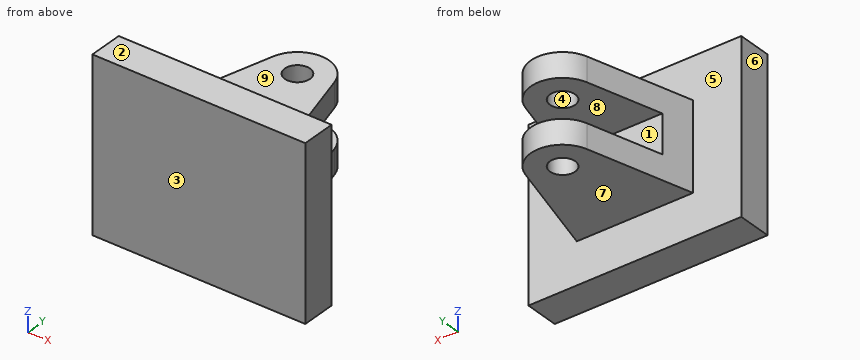
from build123d import *

# Parameters (mm, degrees)
SKETCH3_W               = 100
SKETCH3_H               = 80
BOSS_EXTRUDE2_DEPTH     = 16
BOSS_EXTRUDE3_DEPTH     = 20.5
SKETCH6_R               = 5.911815165
CUT_EXTRUDE1_DEPTH      = 109.559891304
CUT_EXTRUDE2_DEPTH      = 99.615414617
CUT_EXTRUDE2_DEPTH_BACK = 99.615414617
SKETCH8_W               = 18.118513472
SKETCH8_H               = 45.137164109


with BuildPart() as part:
    # Sketch3 → Boss-Extrude2 (new body)
    with BuildSketch(Plane(origin=(0, 0, 0), x_dir=(1, 0, 0), z_dir=(0, 1, 0))):
        Rectangle(SKETCH3_W, SKETCH3_H)
    extrude(amount=BOSS_EXTRUDE2_DEPTH)

    # Sketch5 → Boss-Extrude3 (add, symmetric)
    with BuildSketch(Plane.XY):
        with BuildLine():
            Line((-27.294131566, 16), (-14.434798789, 63.927620339))
            ThreePointArc((-14.434798789, 63.927620339), (0, 75), (14.434798789, 63.927620339))
            Line((14.434798789, 63.927620339), (27.294131566, 16))
            Line((27.294131566, 16), (-27.294131566, 16))
        make_face()
    extrude(amount=BOSS_EXTRUDE3_DEPTH, both=True)

    # Sketch6 → Cut-Extrude1 (cut, through all)
    with BuildSketch(Plane.XY.offset(20.5)):
        with Locations((0, 60.054657736)):
            Circle(SKETCH6_R)
    extrude(amount=-CUT_EXTRUDE1_DEPTH, mode=Mode.SUBTRACT)

    # Sketch8 → Cut-Extrude2 (cut, two sides: drawn at the far end of the back side and taken through both)
    with BuildSketch(Plane(origin=(0, 0, 0), x_dir=(0, 0, -1), z_dir=(1, 0, 0)).offset(-CUT_EXTRUDE2_DEPTH_BACK)):
        with Locations((0, 52.431417946)):
            Rectangle(SKETCH8_W, SKETCH8_H)
    extrude(amount=CUT_EXTRUDE2_DEPTH + CUT_EXTRUDE2_DEPTH_BACK, mode=Mode.SUBTRACT)


solid = part.part
Build history of the part. All positions in model axes, mm. Face numbers are marked on the shaded views. A direction names the side the tool comes from. Give positions to 0.01 mm unless a question says otherwise; leave off trailing zeros. Loops run counter-clockwise (first coordinate to the right, second up) from the corner with the lowest first, then second, coordinate; pieces in that order, holes last. Notation, with made-up numbers: (49.25, 76.25) - (104.25, 76.25) arc R18 cw to (104.25, 102.25) - close; hole circle Ø1 at (89, 17.25). An arc over 180 degrees is marked (long way). Write item = value, one per line. Start each with the question number.
1) Band-saw the part on A-A on x = 0. Give the cut face in (y, z), plus the area to 3 significant figures.
2) Band-saw the part on C-C on z = -18. Give the cut face in (x, y), plus the area to 3 significant figures.
3) Drop flat-ended pins along their axis: pin 1 Ø7 at (x, y) = (0, 60.05) entering from -Z; pin 2 Ø1 at (x, y) = (-11, 62) entering from +Z; pin 3 Ø6 at (y, z) = (60, -21) entering from -X; pin 4 Ø13.5 at (x, y) = (0, 60.05) entering from -Z. Give the stop position or say it passes through.
4) Band-saw the part on D-D on x = 18. Give the cut face in (y, z), plus the area to 3 significant figures.
5) Pull direction Y, two halves, no side cores. Call the marked faces 1, 2, 3 and 4: +Y half, -Y half, draft (parallel to the pull), parting line (faces both ways), or undercut.
6) Tool access for the marked faces 5, 6, 7, 8 and 9: list every direction of +Z, -Z, +X, -X, +Y, -Y with a clear straight run to the whole face (end or side of a thin tool).
7) Band-saw the part on B-B on y = 46. Give the cut face in (x, z).
8) Probe probe 1 along Y at (x, z) = (0, 13); probe 2 along Z at (x, y) = (8.5, 67.5); probe 3 along Y at (x, z) = (36, 25). List the from-to ranges inside material, lowest first. Write a range as from..to.
Final values:
q1.outline = (0, -40) - (16, -40) - (16, -20.5) - (54.14, -20.5) - (54.14, -9.06) - (29.86, -9.06) - (29.86, 9.06) - (54.14, 9.06) - (54.14, 20.5) - (16, 20.5) - (16, 40) - (0, 40) - close; (65.97, -20.5) - (75, -20.5) - (75, -9.06) - (65.97, -9.06) - close; (65.97, 9.06) - (75, 9.06) - (75, 20.5) - (65.97, 20.5) - close
q1.area = 2,610 mm²
q2.outline = (-50, 0) - (50, 0) - (50, 16) - (27.29, 16) - (14.43, 63.93) arc R14.95 ccw to (-14.43, 63.93) - (-27.29, 16) - (-50, 16) - close; hole circle Ø11.82 at (0, 60.05)
q2.area = 3,730 mm²
q3.pin_1 = through
q3.pin_2 = 20.5
q3.pin_3 = -16.28
q3.pin_4 = -20.5
q4.outline = (0, -40) - (16, -40) - (16, -20.5) - (50.64, -20.5) - (50.64, -9.06) - (29.86, -9.06) - (29.86, 9.06) - (50.64, 9.06) - (50.64, 20.5) - (16, 20.5) - (16, 40) - (0, 40) - close
q4.area = 2,320 mm²
q5.face_1 = +Y half
q5.face_2 = draft
q5.face_3 = -Y half
q5.face_4 = undercut
q6.face_5 = +Y
q6.face_6 = +Z, -Z, -X, +Y, -Y
q6.face_7 = -Z, +X, -X, +Y
q6.face_8 = +X, -X, +Y
q6.face_9 = +Z, +X, -X, +Y
q7.outline = (-19.24, -20.5) - (19.24, -20.5) - (19.24, -9.06) - (-19.24, -9.06) - close; (-19.24, 9.06) - (19.24, 9.06) - (19.24, 20.5) - (-19.24, 20.5) - close
q8.probe_1 = 0..54.14, 65.97..75
q8.probe_2 = -20.5..-9.06, 9.06..20.5
q8.probe_3 = 0..16
